```python
from build123d import *

# Parameters (mm, degrees)
F0_W     = 2000
F0_H     = 1000
F1_DEPTH = 25
F2_W     = 100
F2_H     = 100
F3_DEPTH = 725


with BuildPart() as f1:
    # F0 (on Top) → F1 (new body)
    with BuildSketch(Plane.XY):
        with Locations((719.687551, -103.809536)):
            Rectangle(F0_W, F0_H)
    extrude(amount=F1_DEPTH)

    # F2 (on face) → F3 (join)
    with BuildSketch(Plane(origin=(0, 0, 0), x_dir=(1, 0, 0), z_dir=(0, 0, -1))):
        with Locations((-180.312449, 503.809536)):
            Rectangle(F2_W, F2_H)
        with Locations((-180.312449, -296.190464)):
            Rectangle(F2_W, F2_H)
        with Locations((1619.687551, 503.809536)):
            Rectangle(F2_W, F2_H)
        with Locations((1619.687551, -296.190464)):
            Rectangle(F2_W, F2_H)
    extrude(amount=F3_DEPTH)


solid = f1.part
```
Input: part model. Units: mm. Frame: model coordinates. A direction names the side the tool comes from. Give positions to 0.01 mm unless a question says otherwise; leave off trailing zeros. Loops run counter-clockwise (first coordinate to the right, second up) from the corner with the lowest first, then second, coordinate; pieces in that order, holes last. Notation, with made-up numbers: M -28.75,-37 L -5.75,-37 A30 ccw -5.75,-3 Z; hole C 45.25,69.5 d4. An arc over 180 degrees is marked long. Answer as CSV lines item,"result". Start each with the question number.
1. Section A-A on z = -345.5. Return loops of the section in (x, y).
2. Line query: L1, parallel to X at y = 283, z = -204.5; L2, parallel to Z at x = 293, y = 72. Output: solid intervals per line, ascending.
3. Pin query (flat end, axial travel): P1, Ø12, axis at x = 1255, y = 54.5, coming from the -Z side. Return the tip coordinate at first contact, or that it passes through.
4. Reachability of faces 4 (the face through (1669.688, 297, -357)), 5 (the face through (-181, 246.19, -357)), 6 (the face through (-181, -553.81, -357)), 7 (the face through (-230.312, 297, -357)), 8 (the face through (-130.312, -503, -357)) from +Z, -Z, +X, -X, +Y, -Y: full face, straight path, thin tool, end or side. Return the list, or none.
5. Section D-D on y = -348. Return loops of the section in (x, z).
6. Section B-B on y = -486. Return loops of the section in (x, z).
7. Pull-direction query (Y, two-part tool) for faces 1 (the face through (1619, -553.81, -357)), 2 (the face through (1619, -453.81, -357)), 3 (the face through (1619, 346.19, -357)); classes: released by +Y, released by -Y, zero draft, split by the parting line, or undercut.
8. Section C-C on x = 1090. Return loops of the section in (y, z), plus the area to 3 significant figures.
Computed values:
1,outline,"M -230.31,-553.81 L -130.31,-553.81 L -130.31,-453.81 L -230.31,-453.81 Z; M -230.31,246.19 L -130.31,246.19 L -130.31,346.19 L -230.31,346.19 Z; M 1569.69,-553.81 L 1669.69,-553.81 L 1669.69,-453.81 L 1569.69,-453.81 Z; M 1569.69,246.19 L 1669.69,246.19 L 1669.69,346.19 L 1569.69,346.19 Z"
2,L1,"x = -230.31 to -130.31, 1569.69 to 1669.69"
2,L2,"z = 0 to 25"
3,P1,"stops at z = 0"
4,face 4,"-Z, +X, +Y, -Y"
4,face 5,"-Z, +X, -X"
4,face 6,"-Z, +X, -X, -Y"
4,face 7,"-Z, -X, +Y, -Y"
4,face 8,"-Z, +Y, -Y"
5,outline,"M -280.31,0 L 1719.69,0 L 1719.69,25 L -280.31,25 Z"
6,outline,"M -280.31,0 L -230.31,0 L -230.31,-725 L -130.31,-725 L -130.31,0 L 1569.69,0 L 1569.69,-725 L 1669.69,-725 L 1669.69,0 L 1719.69,0 L 1719.69,25 L -280.31,25 Z"
7,face 1,"released by -Y"
7,face 2,"undercut"
7,face 3,"released by +Y"
8,outline,"M -603.81,0 L 396.19,0 L 396.19,25 L -603.81,25 Z"
8,area,"25,000 mm²"
